Job drawing, mm, ordinate dimensions from the low corner. One solid piece. Coordinates: 2 decimals unless noted, no trailing zeros. Write each loop counter-clockwise with the first axis right and the second up, starting at its lowest first coordinate (ties: lowest second). Pieces come first, ordered by that corner, then holes. Notation, with made-up numbers: M 30.25,75.25 L 89.25,75.25 A9 cw 89.25,89.25 Z; hole C 35.5,34 d3. An arc over 180 degrees is marked long. Answer as CSV lines item,"result". Start each with the question number.
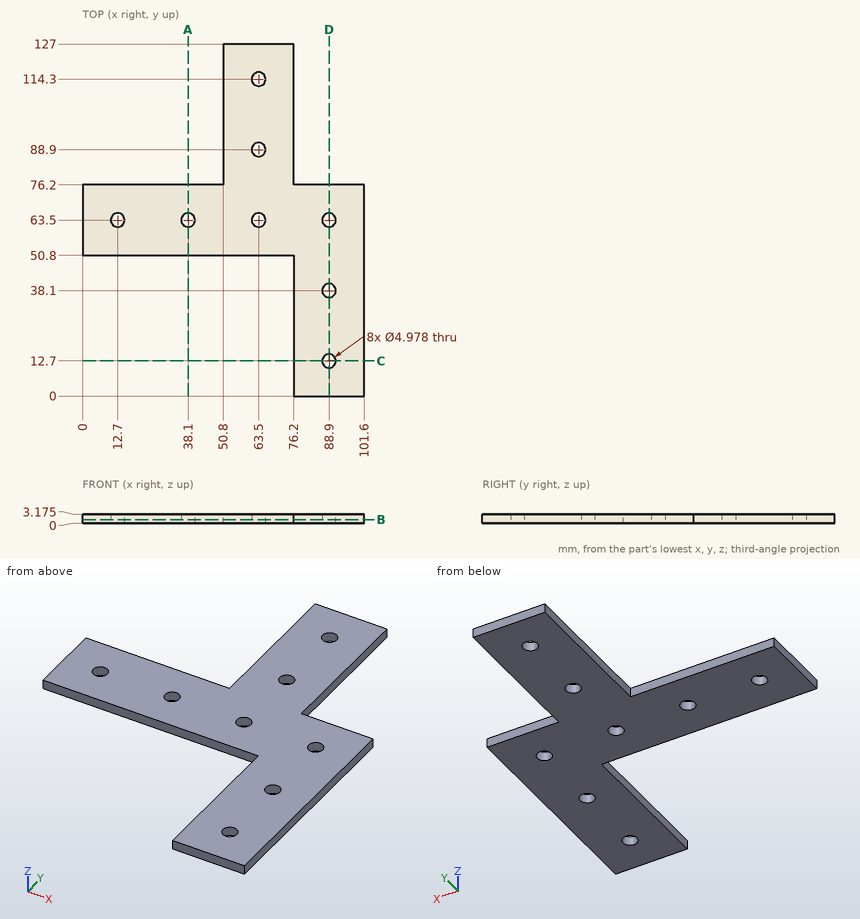
1) Probe L1, parallel to Y at x = 88.9, z = 2.1; L2, parallel to Y at x = 63.5, z = 2.4; L3, parallel to Y at x = 30, z = 2.9. List the from-to ranges inside material, lowest first. Write a range as [from, to].
2) Band-saw the part on C-C, the plane y = 12.7. List the corners of the cut face in (x, z) (1 decimal).
3) Band-saw the part on A-A, the plane x = 38.1. List the corners of the cut face in (y, z) (1 decimal).
4) Pin check, flat tips, straight feed: P1, Ø1, axis at x = 18.5, z = 1, coming from the +Y side; P2, Ø3, axis at x = 12.7, y = 63.5, coming from the -Z side; P3, Ø8, axis at x = 88.9, y = 38.1, coming from the +Z side (3 decimals). Stop position of each tip, or through.
5) Band-saw the part on B-B, the plane z = 1.25. State how many separate pieces and enclosed holes the cut face has, plus the area to 3 significant figures.
6) Band-saw the part on D-D, the plane x = 88.9. List the corners of the cut face in (y, z) (1 decimal).
Result sheet:
1,L1,"y = [0, 10.21], [15.19, 35.61], [40.59, 61.01], [65.99, 76.2]"
1,L2,"y = [50.8, 61.01], [65.99, 86.41], [91.39, 111.81], [116.79, 127]"
1,L3,"y = [50.8, 76.2]"
2,outline,"M 76.2,0 L 86.4,0 L 86.4,3.2 L 76.2,3.2 Z; M 91.4,0 L 101.6,0 L 101.6,3.2 L 91.4,3.2 Z"
3,outline,"M 50.8,0 L 61,0 L 61,3.2 L 50.8,3.2 Z; M 66,0 L 76.2,0 L 76.2,3.2 L 66,3.2 Z"
4,P1,"stops at y = 76.2"
4,P2,"passes through"
4,P3,"stops at z = 3.175"
5,separate pieces,"1"
5,enclosed holes,"8"
5,area,"5,010 mm²"
6,outline,"M 0,0 L 10.2,0 L 10.2,3.2 L 0,3.2 Z; M 15.2,0 L 35.6,0 L 35.6,3.2 L 15.2,3.2 Z; M 40.6,0 L 61,0 L 61,3.2 L 40.6,3.2 Z; M 66,0 L 76.2,0 L 76.2,3.2 L 66,3.2 Z"
